Check sheet for the modelled part. Datum: model origin and axes. Units: mm. A direction names the side the tool comes from. Round coordinates to 2 decimals unless told otherwise and drop trailing zeros. Loops run counter-clockwise (first coordinate to the right, second up) from the corner with the lowest first, then second, coordinate; pieces in that order, holes last. Notation, with made-up numbers: M 39.25,74 L 63.25,74 A16 cw 63.25,78 Z; hole C -18.75,29.25 d7. An arc over 180 degrees is marked long. Write item = value, one per line. Start each with the question number.
(1) Go/stop test with flat-tipped pins: P1, Ø1.5, axis at x = 218.5, z = 1.5, coming from the +Y side; P2, Ø1.5, axis at x = 218, z = 1.5, coming from the -Y side; P3, Ø1.5, axis at y = 133.5, z = 1, coming from the +X side; P4, Ø1.8, axis at x = 191.25, y = 194.1, coming from the +Z side. Record where each tip stops, or that it passes through.
(2) Mould release check, pull along X, two halves, no side actions. Record for faces 1 (the face through (26.19, 178.5, 1.52)), 2 (the face through (35, 185, 0)): pulls with the +X half, pulls with the -X half, needs draft (parallel to the pull), parting line crosses it, or undercut.
(3) Cross-section at B-B on y = 185.6. Record the boundary of the cut face in (x, z), plus the area to 3 significant figures.
(4) Scan lines: L1, parallel to Y at x = 46, z = 2.15; L2, parallel to X at y = 194.1, z = 1.4; L3, parallel to Y at x = 31.25, z = 1.25. Record each from-to range of solid material in increasing order. Write a range as from..to.
(5) Set-up check for faces 3 (the face through (203.69, 178.5, 1.52)), 4 (the face through (176, 156, 2)): record each of +Z, -Z, +X, -X, +Y, -Y from which the full face is reachable in a straight line by a thin tool's end or side.
(6) Cross-section at C-C on z = 1.5. State how many separate pieces and enclosed holes the cut face has, plus the area to 3 significant figures.
(7) Cross-section at A-A on x = 129.5. Record the boundary of the cut face in (y, z).
from build123d import *

# Parameters (mm, degrees)
SKETCH_W        = 220
SKETCH_H        = 300
SKETCH_W_2      = 129
SKETCH_H_2      = 229
PAD_DEPTH       = 3
SKETCH001_W     = 143
SKETCH001_H     = 237
SKETCH001_W_2   = 129
SKETCH001_H_2   = 229
POCKET_DEPTH    = 2
SKETCH002_R     = 8
SKETCH002_R_2   = 1
SKETCH002_R_3   = 3.6
SKETCH002_W     = 3.8
SKETCH002_H     = 10.4
SKETCH002_W_2   = 20
SKETCH002_H_2   = 3
SKETCH002_W_3   = 3
SKETCH002_H_3   = 17
SKETCH002_H_4   = 20
POCKET001_DEPTH = 3.001
SKETCH003_R     = 1
POCKET002_DEPTH = 5


with BuildPart() as part:
    # Sketch → Pad (new body)
    with BuildSketch(Plane.XY):
        with Locations((110, 150)):
            Rectangle(SKETCH_W, SKETCH_H)
        with Locations((110, 129.5)):
            Rectangle(SKETCH_W_2, SKETCH_H_2, mode=Mode.SUBTRACT)
    extrude(amount=PAD_DEPTH)

    # Sketch001 (on Face9 of Pad) → Pocket (cut)
    with BuildSketch(Plane(origin=(0, 0, 0), x_dir=(1, 0, 0), z_dir=(0, 0, -1))):
        with Locations((113, -130.5)):
            Rectangle(SKETCH001_W, SKETCH001_H)
        with Locations((110, -129.5)):
            Rectangle(SKETCH001_W_2, SKETCH001_H_2, mode=Mode.SUBTRACT)
    extrude(amount=-POCKET_DEPTH, mode=Mode.SUBTRACT)

    # Sketch002 (on Face5 of Pocket) → Pocket001 (cut, through all)
    with BuildSketch(Plane.XY.offset(3)):
        with Locations((22.5, 185.6)):
            Circle(SKETCH002_R)
        with Locations((22.5, 160.1)):
            Circle(SKETCH002_R)
        with Locations((13.75, 151.5)):
            Circle(SKETCH002_R_2)
        with Locations((31.25, 151.5)):
            Circle(SKETCH002_R_2)
        with Locations((13.75, 194.1)):
            Circle(SKETCH002_R_2)
        with Locations((31.25, 194.1)):
            Circle(SKETCH002_R_2)
        with Locations((200, 185.6)):
            Circle(SKETCH002_R)
        with Locations((200, 160.1)):
            Circle(SKETCH002_R)
        with Locations((191.25, 151.6)):
            Circle(SKETCH002_R_2)
        with Locations((208.75, 151.6)):
            Circle(SKETCH002_R_2)
        with Locations((191.25, 194.1)):
            Circle(SKETCH002_R_2)
        with Locations((208.75, 194.1)):
            Circle(SKETCH002_R_2)
        with Locations((107.5, 274.5)):
            Circle(SKETCH002_R_3)
        with Locations((107.5, 264)):
            Circle(SKETCH002_R_2)
        with Locations((120, 264)):
            Circle(SKETCH002_R_2)
        with Locations((107.5, 285)):
            Circle(SKETCH002_R_2)
        with Locations((120, 285)):
            Circle(SKETCH002_R_2)
        with Locations((14.95, 172.95)):
            Rectangle(SKETCH002_W, SKETCH002_H)
        with Locations((206.85, 173.05)):
            Rectangle(SKETCH002_W, SKETCH002_H)
        with Locations((10, 1.5)):
            Rectangle(SKETCH002_W_2, SKETCH002_H_2)
        with Locations((50, 1.5)):
            Rectangle(SKETCH002_W_2, SKETCH002_H_2)
        with Locations((90, 1.5)):
            Rectangle(SKETCH002_W_2, SKETCH002_H_2)
        with Locations((130, 1.5)):
            Rectangle(SKETCH002_W_2, SKETCH002_H_2)
        with Locations((170, 1.5)):
            Rectangle(SKETCH002_W_2, SKETCH002_H_2)
        with Locations((210, 1.5)):
            Rectangle(SKETCH002_W_2, SKETCH002_H_2)
        with Locations((10, 298.5)):
            Rectangle(SKETCH002_W_2, SKETCH002_H_2)
        with Locations((50, 298.5)):
            Rectangle(SKETCH002_W_2, SKETCH002_H_2)
        with Locations((90, 298.5)):
            Rectangle(SKETCH002_W_2, SKETCH002_H_2)
        with Locations((130, 298.5)):
            Rectangle(SKETCH002_W_2, SKETCH002_H_2)
        with Locations((170, 298.5)):
            Rectangle(SKETCH002_W_2, SKETCH002_H_2)
        with Locations((210, 298.5)):
            Rectangle(SKETCH002_W_2, SKETCH002_H_2)
        with Locations((1.5, 11.51)):
            Rectangle(SKETCH002_W_3, SKETCH002_H_3)
        with Locations((1.5, 286.99)):
            Rectangle(SKETCH002_W_3, SKETCH002_H_4)
        with Locations((1.5, 50)):
            Rectangle(SKETCH002_W_3, SKETCH002_H_4)
        with Locations((1.5, 90)):
            Rectangle(SKETCH002_W_3, SKETCH002_H_4)
        with Locations((1.5, 130)):
            Rectangle(SKETCH002_W_3, SKETCH002_H_4)
        with Locations((1.5, 170)):
            Rectangle(SKETCH002_W_3, SKETCH002_H_4)
        with Locations((1.5, 210)):
            Rectangle(SKETCH002_W_3, SKETCH002_H_4)
        with Locations((1.5, 250)):
            Rectangle(SKETCH002_W_3, SKETCH002_H_4)
        with Locations((218.5, 50)):
            Rectangle(SKETCH002_W_3, SKETCH002_H_4)
        with Locations((218.5, 90)):
            Rectangle(SKETCH002_W_3, SKETCH002_H_4)
        with Locations((218.5, 130)):
            Rectangle(SKETCH002_W_3, SKETCH002_H_4)
        with Locations((218.5, 170)):
            Rectangle(SKETCH002_W_3, SKETCH002_H_4)
        with Locations((218.5, 210)):
            Rectangle(SKETCH002_W_3, SKETCH002_H_4)
        with Locations((218.5, 250)):
            Rectangle(SKETCH002_W_3, SKETCH002_H_4)
        with Locations((218.5, 288.49)):
            Rectangle(SKETCH002_W_3, SKETCH002_H_3)
        with Locations((218.5, 11.51)):
            Rectangle(SKETCH002_W_3, SKETCH002_H_3)
    extrude(amount=-POCKET001_DEPTH, mode=Mode.SUBTRACT)

    # Sketch003 (on Face2 of Pocket001) → Pocket002 (cut)
    with BuildSketch(Plane(origin=(0, 0, 0), x_dir=(1, 0, 0), z_dir=(0, 0, -1))):
        with Locations((38.5, -17)):
            Circle(SKETCH003_R)
        with Locations((46, -9.5)):
            Circle(SKETCH003_R)
        with Locations((180, -251.5)):
            Circle(SKETCH003_R)
        with Locations((187.5, -244)):
            Circle(SKETCH003_R)
        with Locations((180, -9.5)):
            Circle(SKETCH003_R)
        with Locations((187.5, -17)):
            Circle(SKETCH003_R)
        with Locations((38.5, -244)):
            Circle(SKETCH003_R)
        with Locations((46, -251.5)):
            Circle(SKETCH003_R)
    extrude(amount=-POCKET002_DEPTH, mode=Mode.SUBTRACT)


solid = part.part
Result:
q1.P1 = 297
q1.P2 = 3
q1.P3 = 217
q1.P4 = through
q2.face_1 = undercut
q2.face_2 = needs draft
q3.outline = M 0,0 L 14.5,0 L 14.5,3 L 0,3 Z; M 30.5,0 L 41.5,0 L 41.5,2 L 45.5,2 L 45.5,3 L 30.5,3 Z; M 174.5,2 L 184.5,2 L 184.5,0 L 192,0 L 192,3 L 174.5,3 Z; M 208,0 L 220,0 L 220,3 L 208,3 Z
q3.area = 149 mm^2
q4.L1 = 3..8.5, 10.5..15, 244..250.5, 252.5..297
q4.L2 = 0..12.75, 14.75..30.25, 32.25..41.5, 184.5..190.25, 192.25..207.75, 209.75..220
q4.L3 = 0..150.5, 152.5..193.1, 195.1..300
q5.face_3 = +Z, -Z
q5.face_4 = -Z
q6.separate_pieces = 1
q6.enclosed_holes = 28
q6.area = 29,500 mm^2
q7.outline = M 3,0 L 12,0 L 12,2 L 15,2 L 15,3 L 3,3 Z; M 244,2 L 249,2 L 249,0 L 297,0 L 297,3 L 244,3 Z
